Design review of the part built by this model. Coordinates are the model's own, in mm. Give positions to 0.01 mm unless a question says otherwise; leave off trailing zeros. Loops run counter-clockwise (first coordinate to the right, second up) from the corner with the lowest first, then second, coordinate; pieces in that order, holes last.
from build123d import *

# Parameters (mm, degrees)
F0_R     = 12.5
F1_DEPTH = 300
F2_R     = 5
F3_DEPTH = 25
F4_SIZE  = 5


with BuildPart() as f1:
    # F0 (on Front) → F1 (new body)
    with BuildSketch(Plane.XZ):
        Circle(F0_R)
    extrude(amount=-F1_DEPTH)

    # F2 (on face) → F3 (cut)
    with BuildSketch(Plane.XZ):
        Circle(F2_R)
    extrude(amount=-F3_DEPTH, mode=Mode.SUBTRACT)

    # F4
    f4_edges = [f1.edges().sort_by_distance(p)[0] for p in [
        (-12.5, 0, 0),
    ]]
    chamfer(f4_edges, length=F4_SIZE)


solid = f1.part
Q1. Draft analysis for pull direction Z (two halves, no side actions). For faces 1 (the face through (-1.08, 12.32, -4.88)), 2 (the face through (0, 25, 0)), 3 (the face through (0, 300, 0)), 4 (the face through (7.385, 0.243, 2.326)), state which applies: pulls with the +Z half, pulls with the -Z half, needs draft (parallel to the pull), parting line crosses it, or undercut.
Results:
face 1: undercut
face 2: undercut
face 3: needs draft
face 4: parting line crosses it
Q2. Take a section at C-C (y = 64.5). Give the boundary of the cut face in (x, z), plus the area to 3 significant figures.
Results:
outline: circle Ø25 at (0, 0)
area: 491 mm2
Q3. Take a section at A-A (x = 0). Give the boundary of the cut face in (y, z).
Results:
outline: (0, -7.5) - (5, -12.5) - (300, -12.5) - (300, 12.5) - (5, 12.5) - (0, 7.5) - (0, 5) - (25, 5) - (25, -5) - (0, -5) - close
Q4. Insertion check: pin 1 (5 mm diameter, centred on x = 7, z = -8.5, fed in from -Y); pin 2 (10 mm diameter, centred on x = 6.5, y = 72.5, fed in from -Z); pin 3 (3 mm diameter, centred on x = -5.5, z = 7.5, fed in from -Y). Each pin has a flat end and moves straight along its axis. Give the tip position at first contact, or say it passes through.
Results:
pin 1: stops at y = 1.01
pin 2: stops at z = -12.41
pin 3: stops at y = 0.3
Q5. Wall thickness on line 1 (Z direction, x = 0, y = 19); line 2 (Y direction, x = -3, z = -3.5); line 3 (X direction, y = 79.5, z = 0.5): over which ranges is each line inside the solid? List them lowest first.
Results:
line 1: z = -12.5 to -5, 5 to 12.5
line 2: y = 25 to 300
line 3: x = -12.49 to 12.49
Q6. Take a section at B-B (z = 0). Give the boundary of the cut face in (x, y), plus the area to 4 significant figures.
Results:
outline: (-12.5, 5) - (-7.5, 0) - (-5, 0) - (-5, 25) - (5, 25) - (5, 0) - (7.5, 0) - (12.5, 5) - (12.5, 300) - (-12.5, 300) - close
area: 7,225 mm2
